Work out the finished part from the listing and answer in its coordinate system (mm). Coordinates: 2 decimals unless noted, no trailing zeros. Write each loop counter-clockwise with the first axis right and the second up, starting at its lowest first coordinate (ties: lowest second). Pieces come first, ordered by that corner, then holes. Notation, with made-up numbers: M 12.5,-17 L 67.5,-17 A19 ccw 67.5,-13 Z; hole C -34,29 d3. An arc over 180 degrees is marked long. Use CSV: the item, a comma, the result in double quotes.
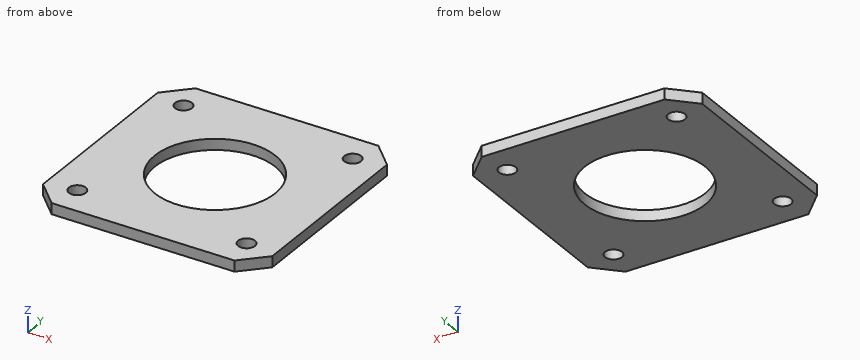
from build123d import *

# Parameters (mm, degrees)
PAD_DEPTH     = 2
SKETCH001_R   = 1.55
SKETCH001_R_2 = 11.05
POCKET_DEPTH  = 5


with BuildPart() as part:
    # Sketch → Pad (new body)
    with BuildSketch(Plane.XY):
        Polygon((21, -16.757359), (21, 16.757359), (16.757359, 21), (-16.757359, 21), (-21, 16.757359), (-21, -16.757359), (-16.757359, -21), (16.757359, -21), align=None)
    extrude(amount=PAD_DEPTH)

    # Sketch001 (on Face10 of Pad) → Pocket (cut)
    with BuildSketch(Plane.XY.offset(2)):
        with Locations((-15.5, 15.5)):
            Circle(SKETCH001_R)
        with Locations((15.5, 15.5)):
            Circle(SKETCH001_R)
        with Locations((15.5, -15.5)):
            Circle(SKETCH001_R)
        with Locations((-15.5, -15.5)):
            Circle(SKETCH001_R)
        Circle(SKETCH001_R_2)
    extrude(amount=-POCKET_DEPTH, mode=Mode.SUBTRACT)


solid = part.part
Item 1: Consider probe 1 along Y at (x, z) = (15.5, 0.7); probe 2 along X at (y, z) = (15, 1); probe 3 along Y at (x, z) = (0, 0.4). Determine where each line is inside the solid, lowest interval first.
Answer:
probe 1,"y = -21 to -17.05, -13.95 to 13.95, 17.05 to 21"
probe 2,"x = -21 to -16.97, -14.03 to 14.03, 16.97 to 21"
probe 3,"y = -21 to -11.05, 11.05 to 21"
Item 2: Given pin 1 (4 mm diameter, centred on x = -15.5, y = -15.5, fed in from +Z), flat-ended and moving along its own axis, determine where the tip first touches the part or whether it passes through.
Answer:
pin 1,"stops at z = 2"
Item 3: The part is cut by section A-A (x = 15.5). Write down the section's boundary in (y, z).
Answer:
outline,"M -21,0 L -17.05,0 L -17.05,2 L -21,2 Z; M -13.95,0 L 13.95,0 L 13.95,2 L -13.95,2 Z; M 17.05,0 L 21,0 L 21,2 L 17.05,2 Z"
Item 4: The part is cut by section D-D (y = -3). Write down the section's boundary in (x, z).
Answer:
outline,"M -21,0 L -10.63,0 L -10.63,2 L -21,2 Z; M 10.63,0 L 21,0 L 21,2 L 10.63,2 Z"
Item 5: The part is cut by section C-C (x = 0). Write down the section's boundary in (y, z).
Answer:
outline,"M -21,0 L -11.05,0 L -11.05,2 L -21,2 Z; M 11.05,0 L 21,0 L 21,2 L 11.05,2 Z"
